For this review, take the finished solid that the model builds, in its own axes (mm). Face numbers are marked on the shaded views. Round coordinates to 2 decimals unless told otherwise and drop trailing zeros. Write each loop counter-clockwise with the first axis right and the second up, starting at its lowest first coordinate (ties: lowest second). Pieces come first, ordered by that corner, then holes. Notation, with made-up numbers: (-26, -13) -> (0, -13) arc R24 cw to (0, 0) -> close; hole circle Ø2 at (7, -10). An arc over 180 degrees is marked (long way). Write each question's results on one line, items separated by ' | '. Start each with the question number.
Item 1: Add section A-A (x = 70). State the section outline as (y, z) points, plus the area to 3 significant figures.
Item 2: To check wall thickness, follow line 1 along X through (y, z) = (-2.25, -0.75); line 2 along Y through (x, z) = (48.5, -1.25); line 3 along Y through (x, z) = (90, -5). State the ranges of each line that lie inside material, in increasing order.
Item 3: Add section C-C (x = 50). State the section outline as (y, z) points.
Item 4: The part is to be moulded in two halves that separate along Y. For the marked faces 1, 2 and 3, say which applies: +Y half, -Y half, draft (parallel to the pull), parting line (faces both ways), or undercut.
Item 5: Add section B-B (z = -2.5). Count the separate pieces of the cut face and the enclosed holes in it, plus the area to 3 significant figures.
from build123d import *

# Parameters (mm, degrees)
SKETCH_W   = 100
SKETCH_H   = 10
SKETCH_R   = 1
SKETCH_R_2 = 2
SKETCH_R_3 = 3
SKETCH_R_4 = 4
SKETCH_R_5 = 0.5
SKETCH_R_6 = 1.5
SKETCH_R_7 = 2.5
SKETCH_R_8 = 3.5
SKETCH_R_9 = 4.5
PAD_DEPTH  = 10


with BuildPart() as part:
    # Sketch → Pad (new body)
    with BuildSketch(Plane.XY):
        with Locations((50, 0)):
            Rectangle(SKETCH_W, SKETCH_H)
        with Locations((20, 0)):
            Circle(SKETCH_R, mode=Mode.SUBTRACT)
        with Locations((40, 0)):
            Circle(SKETCH_R_2, mode=Mode.SUBTRACT)
        with Locations((60, 0)):
            Circle(SKETCH_R_3, mode=Mode.SUBTRACT)
        with Locations((80, 0)):
            Circle(SKETCH_R_4, mode=Mode.SUBTRACT)
        with Locations((10, 0)):
            Circle(SKETCH_R_5, mode=Mode.SUBTRACT)
        with Locations((30, 0)):
            Circle(SKETCH_R_6, mode=Mode.SUBTRACT)
        with Locations((50, 0)):
            Circle(SKETCH_R_7, mode=Mode.SUBTRACT)
        with Locations((70, 0)):
            Circle(SKETCH_R_8, mode=Mode.SUBTRACT)
        with Locations((90, 0)):
            Circle(SKETCH_R_9, mode=Mode.SUBTRACT)
    extrude(amount=-PAD_DEPTH)


solid = part.part
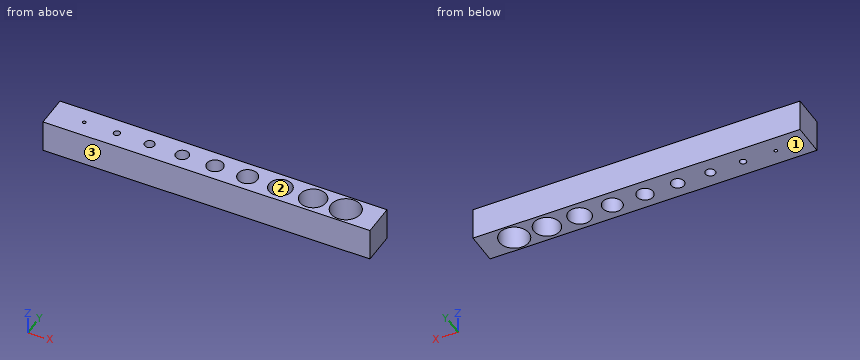
Responses:
1) outline: (-5, -10) -> (-3.5, -10) -> (-3.5, 0) -> (-5, 0) -> close; (3.5, -10) -> (5, -10) -> (5, 0) -> (3.5, 0) -> close | area: 30.0 mm^2
2) line 1: x = 0 to 48.91, 51.09 to 58.02, 61.98 to 67.32, 72.68 to 76.69, 83.31 to 86.1, 93.9 to 100 | line 2: y = -5 to -2, 2 to 5 | line 3: y = -5 to -4.5, 4.5 to 5
3) outline: (-5, -10) -> (-2.5, -10) -> (-2.5, 0) -> (-5, 0) -> close; (2.5, -10) -> (5, -10) -> (5, 0) -> (2.5, 0) -> close
4) face 1: draft | face 2: undercut | face 3: -Y half
5) separate pieces: 1 | enclosed holes: 9 | area: 776 mm^2
